from build123d import *

# Parameters (mm, degrees)
SKETCH1_W           = 65
SKETCH1_H           = 56
BOSS_EXTRUDE1_DEPTH = 3.175
SKETCH2_R           = 1.190625
SKETCH2_W           = 6.35
SKETCH2_H           = 3.175
CUT_EXTRUDE1_DEPTH  = 3.175
FILLET1_R           = 1.5875
SKETCH3_R           = 3.106099532
CUT_EXTRUDE2_DEPTH  = 3.175


with BuildPart() as part:
    # Sketch1 → Boss-Extrude1 (new body)
    with BuildSketch(Plane(origin=(0, 0, 0), x_dir=(1, 0, 0), z_dir=(0, 1, 0))):
        with Locations((32.5, 28)):
            Rectangle(SKETCH1_W, SKETCH1_H)
    extrude(amount=BOSS_EXTRUDE1_DEPTH)

    # Sketch2 → Cut-Extrude1 (cut)
    with BuildSketch(Plane(origin=(0, 3.175, 0), x_dir=(1, 0, 0), z_dir=(0, 1, 0))):
        with Locations((62, 53)):
            Circle(SKETCH2_R)
        with Locations((3, 53)):
            Circle(SKETCH2_R)
        with Locations((3, 3)):
            Circle(SKETCH2_R)
        with Locations((62, 3)):
            Circle(SKETCH2_R)
        with Locations((13.45, 32.7625)):
            Rectangle(SKETCH2_W, SKETCH2_H)
        with Locations((38.85, 32.7625)):
            Rectangle(SKETCH2_W, SKETCH2_H)
        with Locations((51.55, 32.7625)):
            Rectangle(SKETCH2_W, SKETCH2_H)
        with Locations((26.15, 32.7625)):
            Rectangle(SKETCH2_W, SKETCH2_H)
        with Locations((26.15, 23.2375)):
            Rectangle(SKETCH2_W, SKETCH2_H)
        with Locations((13.45, 23.2375)):
            Rectangle(SKETCH2_W, SKETCH2_H)
        with Locations((51.55, 23.2375)):
            Rectangle(SKETCH2_W, SKETCH2_H)
        with Locations((38.85, 23.2375)):
            Rectangle(SKETCH2_W, SKETCH2_H)
    extrude(amount=-CUT_EXTRUDE1_DEPTH, mode=Mode.SUBTRACT)

    # Fillet1
    fillet1_edges = [part.edges().sort_by_distance(p)[0] for p in [
        (0, 1.5875, -56),
        (65, 1.5875, -56),
        (65, 1.5875, 0),
        (0, 1.5875, 0),
    ]]
    fillet(fillet1_edges, radius=FILLET1_R)

    # Sketch3 → Cut-Extrude2 (cut)
    with BuildSketch(Plane(origin=(0, 3.175, 0), x_dir=(1, 0, 0), z_dir=(0, 1, 0))):
        with Locations((5.068, 28)):
            Circle(SKETCH3_R)
        with Locations((59.932, 28)):
            Circle(SKETCH3_R)
    extrude(amount=-CUT_EXTRUDE2_DEPTH, mode=Mode.SUBTRACT)


solid = part.part
Work out the finished part from the listing and answer in its coordinate system (mm). A direction names the side the tool comes from. Give positions to 0.01 mm unless a question says otherwise; leave off trailing zeros. Order: outer loops, then holes, each group sorted by start corner. A loop starts at its lowest first (then second) coordinate and runs counter-clockwise, first axis right, second up. Notation, with made-up numbers: (69, 44) -> (83, 44) arc R23 ccw to (83, 59) -> close; hole circle Ø7 at (-3, 44.5). An arc over 180 degrees is marked (long way). One line per item, written item: value.
Item 1: Determine the mould class of faces 1 (the cylindrical face through (64.52, 1.61, -0.45)), 2 (the flat face through (42.025, 2, -33)), 3 (the flat face through (65, 2, -28)) for opening direction Z: released by +Z, released by -Z, zero draft, split by the parting line, or undercut.
Answer sheet:
face 1: released by +Z
face 2: undercut
face 3: zero draft
Item 2: Find section B-B, the plane x = 38.5. Give the vertices of the cut face in (y, z) (3 decimals), plus the area to 3 significant figures.
Answer sheet:
outline: (0, -56) -> (3.175, -56) -> (3.175, -34.35) -> (0, -34.35) -> close; (0, -31.175) -> (3.175, -31.175) -> (3.175, -24.825) -> (0, -24.825) -> close; (0, -21.65) -> (3.175, -21.65) -> (3.175, 0) -> (0, 0) -> close
area: 158 mm²
Item 3: Straight lines are drawn through the part: probe 1 along Z at (x, y) = (14.5, 0.25) (3 decimals); probe 2 along X at (y, z) = (1.9, -3); probe 3 along X at (y, z) = (1.4, -28). For each, find the intervals that lie inside material, in ascending order.
Answer sheet:
probe 1: -56 to -34.35, -31.175 to -24.825, -21.65 to 0
probe 2: 0 to 1.81, 4.19 to 60.81, 63.19 to 65
probe 3: 0 to 1.96, 8.17 to 56.83, 63.04 to 65
Item 4: A tool of negligible diameter and unlimited length cuts with its end or side. For faces 4 (the flat face through (32, 2, -56)), 5 (the flat face through (52, 2, -21.65)), from which of +Z, -Z, +X, -X, +Y, -Y can it reach the whole face along a straight path? Write none if from no direction.
Answer sheet:
face 4: -Z, +X, -X, +Y, -Y
face 5: +Y, -Y
Item 5: Find section A-A, the plane z = -3. Give the vertices of the cut face in (x, y) (3 decimals), plus the area to 3 significant figures.
Answer sheet:
outline: (0, 0) -> (1.809, 0) -> (1.809, 3.175) -> (0, 3.175) -> close; (4.191, 0) -> (60.809, 0) -> (60.809, 3.175) -> (4.191, 3.175) -> close; (63.191, 0) -> (65, 0) -> (65, 3.175) -> (63.191, 3.175) -> close
area: 191 mm²
Item 6: Find section C-C, the plane x = 62. Give the vertices of the cut face in (y, z) (3 decimals), plus the area to 3 significant figures.
Answer sheet:
outline: (0, -56) -> (3.175, -56) -> (3.175, -54.191) -> (0, -54.191) -> close; (0, -51.809) -> (3.175, -51.809) -> (3.175, -30.318) -> (0, -30.318) -> close; (0, -25.682) -> (3.175, -25.682) -> (3.175, -4.191) -> (0, -4.191) -> close; (0, -1.809) -> (3.175, -1.809) -> (3.175, 0) -> (0, 0) -> close
area: 148 mm²
Item 7: Find section D-D, the plane y = 1.95. State how many separate pieces and enclosed holes the cut face has, plus the area to 3 significant figures.
Answer sheet:
separate pieces: 1
enclosed holes: 14
area: 3,400 mm²
